The model under review builds one solid part; all positions refer to its coordinate system, in mm. A direction names the side the tool comes from. Coordinates: 2 decimals unless noted, no trailing zeros. Write item = value, one per line. Start each with the question number.
Q1. Clearance check with a flat-ended pin moving along its axis: pin 1 Ø8 at (x, y) = (0, 0) entering from +Z (3 decimals). State where the tip first meets the part, or that it passes through.
Q2. For faces 4 (the face through (-7.5, 0, 2)), 5 (the face through (3.32, 0.74, -138.71)), 6 (the face through (3.32, 0.74, 138.71)), list the 3-axis set-ups (+Z, -Z, +X, -X, +Y, -Y) from which the entire face can be reached by the end or side of a thin tool; tool diameter is ignored.
Q3. Wall thickness on probe 1 along X at (y, z) = (0, -136.5); probe 2 along Z at (x, y) = (3.25, -0.25): over which ranges is each line inside the solid? List them lowest first.
Q4. Mouldability with a two-part tool opening along Y and no side actions: class faces 1 (the face through (0, -7.5, 2)), 2 (the face through (0.359, 0.469, -126.062)), 3 (the face through (-3, 3, 150)) as released by +Y, released by -Y, zero draft, split by the parting line, or undercut.
from build123d import *

# Parameters (mm, degrees)
SKETCH1_W           = 15
SKETCH1_H           = 15
BOSS_EXTRUDE1_DEPTH = 150


with BuildPart() as part:
    # Sketch1 → Boss-Extrude1 (new, symmetric)
    with BuildSketch(Plane.XY):
        Rectangle(SKETCH1_W, SKETCH1_H)
    extrude(amount=BOSS_EXTRUDE1_DEPTH, both=True)

    # Sketch3 → M8 Tapped Hole1 (revolve, cut)
    with BuildSketch(Plane(origin=(0, 0, 150), x_dir=(0, -1, 0), z_dir=(1, 0, 0))):
        Polygon((0, 0), (0, 24.292926105), (3.4, 22.25), (3.4, 0.625), (4.025, 0), align=None)
    m8_tapped_hole1 = revolve(axis=Axis((0, 0, 156.35), (0, 0, -1)), mode=Mode.SUBTRACT)

    # Mirror1: M8 Tapped Hole1 across plane
    add(m8_tapped_hole1.mirror(Plane.XY), mode=Mode.SUBTRACT)


solid = part.part
Returned:
q1.pin_1 = 149.975
q2.face_4 = +Z, -Z, -X, +Y, -Y
q2.face_5 = -Z
q2.face_6 = +Z
q3.probe_1 = -7.5 to -3.4, 3.4 to 7.5
q3.probe_2 = -127.67 to 127.67
q4.face_1 = released by -Y
q4.face_2 = undercut
q4.face_3 = zero draft
